Geometry check sheet. Reference: the model listing, model coordinates, mm. A direction names the side the tool comes from. Coordinates: 2 decimals unless noted, no trailing zeros. Write each loop counter-clockwise with the first axis right and the second up, starting at its lowest first coordinate (ties: lowest second). Pieces come first, ordered by that corner, then holes.
from build123d import *

# Parameters (mm, degrees)
SKETCH1_W                 = 30
SKETCH1_H                 = 10
BOSS_EXTRUDE1_DEPTH       = 90
M4X0_7_TAPPED_HOLE1_D     = 3.3
M4X0_7_TAPPED_HOLE1_DEPTH = 15
M4X0_7_TAPPED_HOLE1_TIP   = 0.991420021
M4X0_7_TAPPED_HOLE2_D     = 3.3
M4X0_7_TAPPED_HOLE2_DEPTH = 15
M4X0_7_TAPPED_HOLE2_TIP   = 0.991420021
M4X0_7_TAPPED_HOLE3_D     = 3.3
M4_CLEARANCE_HOLE1_D      = 4.5
M4_CLEARANCE_HOLE1_DEPTH  = 15
M4_CLEARANCE_HOLE1_TIP    = 1.351936393
SKETCH13_W                = 8
SKETCH13_H                = 50
CUT_EXTRUDE1_DEPTH        = 8
CHAMFER4_SIZE             = 8
CHAMFER5_SIZE             = 4


# Some blends are built 0.0001 mm under size
with BuildPart() as part:
    # Sketch1 → Boss-Extrude1 (new body)
    with BuildSketch(Plane(origin=(0, 0, 0), x_dir=(1, 0, 0), z_dir=(0, 1, 0))):
        Rectangle(SKETCH1_W, SKETCH1_H)
    extrude(amount=BOSS_EXTRUDE1_DEPTH)

    # M4x0.7 Tapped Hole1
    with Locations(Plane(origin=(0, 0, 0), x_dir=(-1, 0, 0), z_dir=(0, -1, 0))):
        with Locations((-10, 0), (10, 0), (0, 0)):
            Hole(M4X0_7_TAPPED_HOLE1_D / 2, depth=M4X0_7_TAPPED_HOLE1_DEPTH)
            with Locations((0, 0, -(M4X0_7_TAPPED_HOLE1_DEPTH + M4X0_7_TAPPED_HOLE1_TIP / 2))):  # 118° drill point
                Cone(0, M4X0_7_TAPPED_HOLE1_D / 2, M4X0_7_TAPPED_HOLE1_TIP, mode=Mode.SUBTRACT)

    # M4x0.7 Tapped Hole2
    with Locations(Plane(origin=(0, 90, 0), x_dir=(1, 0, 0), z_dir=(0, 1, 0))):
        with Locations((-10, 0), (10, 0)):
            Hole(M4X0_7_TAPPED_HOLE2_D / 2, depth=M4X0_7_TAPPED_HOLE2_DEPTH)
            with Locations((0, 0, -(M4X0_7_TAPPED_HOLE2_DEPTH + M4X0_7_TAPPED_HOLE2_TIP / 2))):  # 118° drill point
                Cone(0, M4X0_7_TAPPED_HOLE2_D / 2, M4X0_7_TAPPED_HOLE2_TIP, mode=Mode.SUBTRACT)

    # M4x0.7 Tapped Hole3 (through all)
    with Locations(Plane.XY.offset(5)):
        with Locations((0, 70), (0, 20)):
            Hole(M4X0_7_TAPPED_HOLE3_D / 2)

    # M4 Clearance Hole1
    with Locations(Plane(origin=(0, 90, 0), x_dir=(1, 0, 0), z_dir=(0, 1, 0))):
        with Locations((0, 0)):
            Hole(M4_CLEARANCE_HOLE1_D / 2, depth=M4_CLEARANCE_HOLE1_DEPTH)
            with Locations((0, 0, -(M4_CLEARANCE_HOLE1_DEPTH + M4_CLEARANCE_HOLE1_TIP / 2))):  # 118° drill point
                Cone(0, M4_CLEARANCE_HOLE1_D / 2, M4_CLEARANCE_HOLE1_TIP, mode=Mode.SUBTRACT)

    # Sketch13 → Cut-Extrude1 (cut)
    with BuildSketch(Plane.ZY.offset(15)):
        with Locations((1, 45)):
            Rectangle(SKETCH13_W, SKETCH13_H)
    extrude(amount=-CUT_EXTRUDE1_DEPTH, mode=Mode.SUBTRACT)

    # Chamfer4
    chamfer4_edges = [part.edges().sort_by_distance(p)[0] for p in [
        (-7, 45, -3),
    ]]
    chamfer(chamfer4_edges, length=CHAMFER4_SIZE - 0.0001)  # a hair under: the kernel refuses the full size

    # Chamfer5
    # the kernel refuses this chamfer: 4 mm, written as the material it takes off along each edge
    with BuildSketch(Plane(origin=(-25.286731952, 20, 5), x_dir=(0, -0.9996219169112968, 0.02749587661058627), z_dir=(1, 0, 0))) as chamfer5_piece_1_section:
        Polygon((CHAMFER5_SIZE * 0.999621916911, CHAMFER5_SIZE * 0.0274958766106), (-CHAMFER5_SIZE * 0.0274958766106, CHAMFER5_SIZE * 0.999621916911), (0, 0), align=None)
    chamfer5_piece_1 = extrude(amount=18.286731952, mode=Mode.PRIVATE)
    chamfer5_piece_1 = split(chamfer5_piece_1, bisect_by=Plane(origin=(-9.899926501, 18.600001, 2.099973499), z_dir=(-0.7071067811865476, 0, 0.7071067811865476)), keep=Keep.TOP, mode=Mode.PRIVATE)
    add(chamfer5_piece_1, mode=Mode.SUBTRACT)
    with BuildSketch(Plane(origin=(-15, 20, -3), x_dir=(-0.027495876610586487, -0.9996219169112968, 0), z_dir=(0, 0, 1))) as chamfer5_piece_2_section:
        Polygon((CHAMFER5_SIZE * 0.999621916911, CHAMFER5_SIZE * 0.0274958766106), (-CHAMFER5_SIZE * 0.0274958766106, CHAMFER5_SIZE * 0.999621916911), (0, 0), align=None)
    chamfer5_piece_2 = extrude(amount=18.286731952, mode=Mode.PRIVATE)
    chamfer5_piece_2 = split(chamfer5_piece_2, bisect_by=Plane(origin=(-12.099973499, 18.600001, -0.100073499), z_dir=(-0.7071067811865476, 0, 0.7071067811865476)), keep=Keep.TOP, mode=Mode.PRIVATE)
    add(chamfer5_piece_2, mode=Mode.SUBTRACT)
    with BuildSketch(Plane(origin=(-25.286731952, 70, 5), x_dir=(0, -0.027495876610585623, -0.9996219169112968), z_dir=(1, 0, 0))) as chamfer5_piece_3_section:
        Polygon((CHAMFER5_SIZE * 0.999621916911, CHAMFER5_SIZE * 0.0274958766106), (-CHAMFER5_SIZE * 0.0274958766106, CHAMFER5_SIZE * 0.999621916911), (0, 0), align=None)
    chamfer5_piece_3 = extrude(amount=18.286731952, mode=Mode.PRIVATE)
    chamfer5_piece_3 = split(chamfer5_piece_3, bisect_by=Plane(origin=(-9.899926501, 71.399999, 2.099973499), z_dir=(-0.7071067811865476, 0, 0.7071067811865476)), keep=Keep.TOP, mode=Mode.PRIVATE)
    add(chamfer5_piece_3, mode=Mode.SUBTRACT)
    with BuildSketch(Plane(origin=(-15, 70, 15.286731952), x_dir=(0.9996219169112968, -0.027495876610585623, 0), z_dir=(0, 0, -1))) as chamfer5_piece_4_section:
        Polygon((CHAMFER5_SIZE * 0.999621916911, -CHAMFER5_SIZE * 0.0274958766106), (-CHAMFER5_SIZE * 0.0274958766106, -CHAMFER5_SIZE * 0.999621916911), (0, 0), align=None)
    chamfer5_piece_4 = extrude(amount=18.286731952, mode=Mode.PRIVATE)
    chamfer5_piece_4 = split(chamfer5_piece_4, bisect_by=Plane(origin=(-12.099973499, 71.399999, -0.100073499), z_dir=(-0.7071067811865476, 0, 0.7071067811865476)), keep=Keep.TOP, mode=Mode.PRIVATE)
    add(chamfer5_piece_4, mode=Mode.SUBTRACT)


solid = part.part
1. Access from +Z, -Z, +X, -X, +Y, -Y to the whole of each face (thin tool, end or side, straight path). Record for faces 1 (the cylindrical face through (-8.476, 7.605, 0.632)), 2 (the flat face through (-15, 44.4, -3.3)), 3 (the flat face through (-13, 18, 1)).
Computed values:
face 1: -Y
face 2: +Z, -Z, -X, +Y, -Y
face 3: +Z, -X
2. Sectioned sample at A-A, the plane y = 8.5. Record the boundary of the cut face in (x, z).
Computed values:
outline: (-15, -5) - (15, -5) - (15, 5) - (-15, 5) - close; hole circle Ø3.3 at (-10, 0); hole circle Ø3.3 at (0, 0); hole circle Ø3.3 at (10, 0)
3. Sectioned sample at C-C, the plane y = 84. Record the boundary of the cut face in (x, z), and give its area (3 significant figures).
Computed values:
outline: (-15, -5) - (15, -5) - (15, 5) - (-15, 5) - close; hole circle Ø3.3 at (-10, 0); hole circle Ø4.5 at (0, 0); hole circle Ø3.3 at (10, 0)
area: 267 mm2
4. Draft check along Z on faces 4 (the cylindrical face through (0.29, 82.4, -2.23)), 5 (the flat face through (-11, 72, 3)), 6 (the flat face through (0, 90, -3)). Enter one of: released by +Z, released by -Z, zero draft, split by the parting line, or undercut.
Computed values:
face 4: undercut
face 5: released by +Z
face 6: zero draft
5. Gauge pin test, flat ends, axial feed: pin 1 Ø3 at (x, z) = (0, 0) entering from +Y; pin 2 Ø2 at (x, z) = (10, 0) entering from -Y; pin 3 Ø2.5 at (x, z) = (0, 0) entering from +Y. Record the tip position at first contact, or that the pin passes through.
Computed values:
pin 1: stops at y = 74.55
pin 2: stops at y = 15.39
pin 3: stops at y = 74.4
6. Thickness scan on line 1 along Z through (x, y) = (-10, 6.5); line 2 along Y through (x, z) = (-0.5, 4.75); line 3 along Y through (x, z) = (1, 1). Record the ranges inside material, lowest first.
Computed values:
line 1: z = -5 to -1.65, 1.65 to 5
line 2: y = 0 to 18.43, 21.57 to 68.43, 71.57 to 90
line 3: y = 15.14 to 18.69, 21.31 to 68.69, 71.31 to 74.5
